Here's the drawing with two shaded views (mm, measured from the low corner). I have some questions. Give positions to 0.01 mm unless a question says otherwise; leave off trailing zeros. Write each loop counter-clockwise with the first axis right and the second up, starting at its lowest first coordinate (ties: lowest second). Pieces come first, ordered by that corner, then holes. Notation, with made-up numbers: (31.5, 11.5) - (40.5, 11.5) arc R14 cw to (40.5, 34.5) - close; hole circle Ø2 at (-9.5, -26.75). An arc over 180 degrees is marked (long way). Use one line per item in the form item = value.
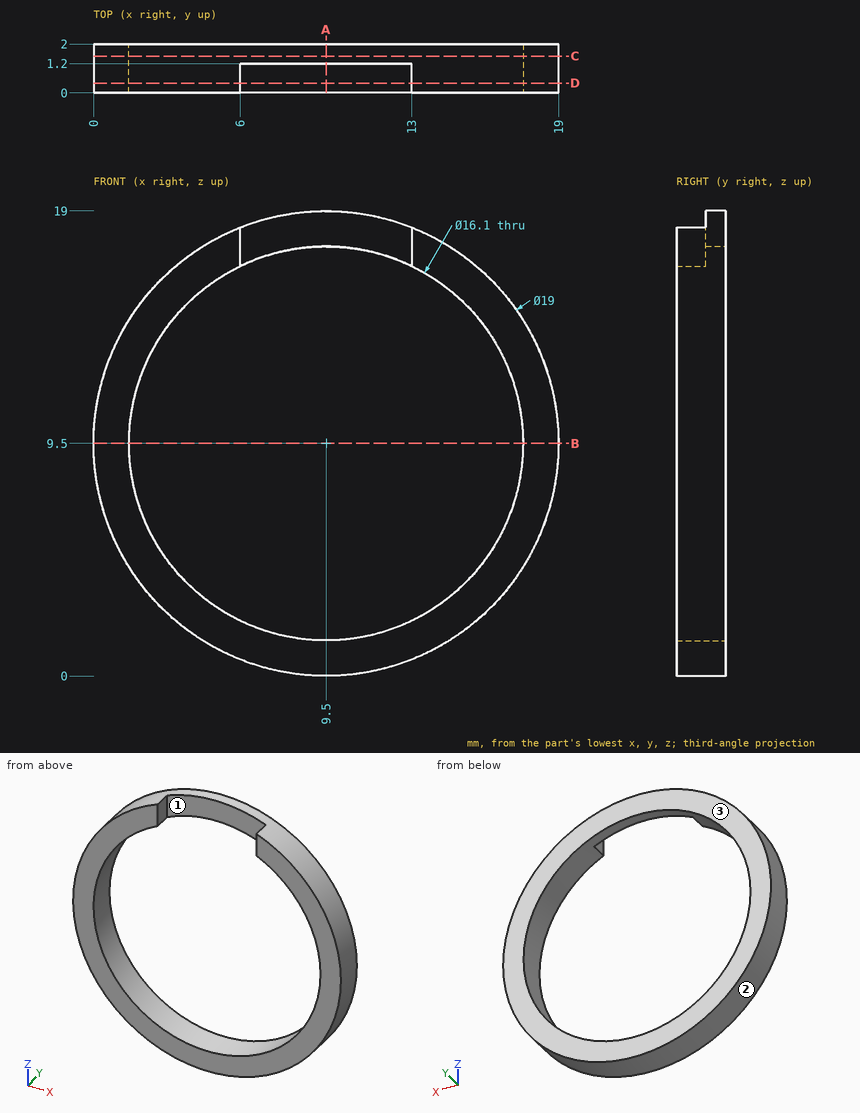
1. Imagine slicing it at A-A, the plane x = 9.5. List the corners of the cut face in (y, z) for me, and give its area (3 significant figures).
Response values:
outline = (0, 0) - (2, 0) - (2, 1.45) - (0, 1.45) - close; (1.2, 17.55) - (2, 17.55) - (2, 19) - (1.2, 19) - close
area = 4.06 mm²
2. Imagine slicing it at B-B, the plane z = 9.5. List the corners of the cut face in (x, y) for me, and give its area (3 significant figures).
Response values:
outline = (0, 0) - (1.45, 0) - (1.45, 2) - (0, 2) - close; (17.55, 0) - (19, 0) - (19, 2) - (17.55, 2) - close
area = 5.80 mm²
3. Imagine slicing it at D-D, the plane y = 0.4. List the corners of the cut face in (x, z) for me.
Response values:
outline = (6, 16.75) - (6, 18.33) arc R9.5 ccw (long way) to (13, 18.33) - (13, 16.75) arc R8.05 cw (long way) to start
4. For pin 1 (0.7 mm diameter, centred on x = 10, z = 18.5, fed in from -Y); pin 2 (1 mm diameter, centred on y = 1, z = 3.5, fed in from -X); pin 3 (1 mm diameter, centred on y = 0.5, z = 18, fed in from +X), each with a flat end and sliding along its axis, tell me the tip position at first contact or that it passes through.
Response values:
pin_1 = 1.2
pin_2 = 1.75
pin_3 = 14.62
5. If I drill on line 1 (X direction, y = 1.4, z = 9.5); line 2 (Z direction, x = 9.5, y = 0.9), over which ranges is the centre line in solid material (lowest first)? Write a range as from..to.
Response values:
line_1 = 0..1.45, 17.55..19
line_2 = 0..1.45
6. Imagine slicing it at C-C, the plane y = 1.5. List the corners of the cut face in (x, z) for me.
Response values:
outline = circle Ø19 at (9.5, 9.5); hole circle Ø16.1 at (9.5, 9.5)
7. If we mould it in two halves opening along X, with no side actions, what happens to the marked faces 1, 2 and 3? For each: pulls with the +X half, pulls with the -X half, needs draft (parallel to the pull), parting line crosses it, or undercut.
Response values:
face_1 = undercut
face_2 = parting line crosses it
face_3 = needs draft
